Autodesk Inventor part; units mm, degrees
ref_plane "YZ Plane" through (0, 0, 0) normal (1, 0, 0) x (0, 1, 0)
ref_plane "XZ Plane" through (0, 0, 0) normal (0, 1, 0) x (-1, 0, 0)
ref_plane "XY Plane" through (0, 0, 0) normal (0, 0, 1) x (1, 0, 0)
sketch "Boceto1" plane through (0, 0, 0) normal (0, 1, 0) x (-1, 0, 0)
  circle A0 centre (0, 0) radius 9
  dimension "d0" = 18
extrude "Extrusión1" add sketch "Boceto1" along normal blind 65
sketch "Boceto2" plane through (0, 65, 0) normal (0, 1, 0) x (1, 0, 0)
  circle A0 centre (0, 0) radius 4.5
  circle A1 centre (0, 0) radius 7
  dimension "d3" = 9
  dimension "d4" = 14
extrude "Extrusión2" cut sketch "Boceto2" against normal blind 0.5
sketch "Boceto3" plane through (0, 0, 0) normal (0, -1, 0) x (1, 0, 0)
  circle A0 centre (0, 0) radius 7
extrude "Extrusión3" cut sketch "Boceto3" against normal blind 0.1
properties part number "Batería"
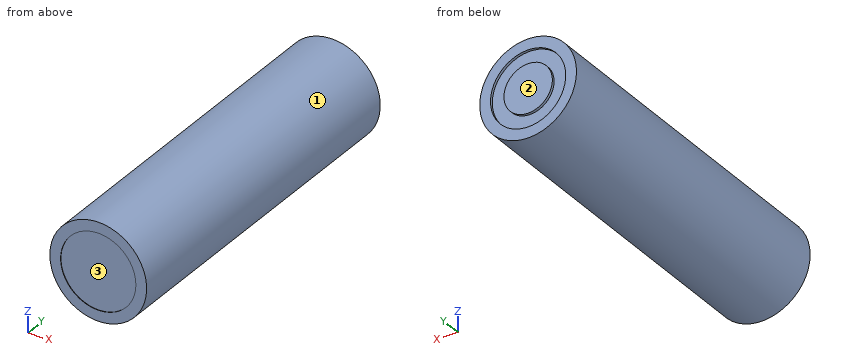
Geometry: final body of the model. Coordinates: model frame, mm. Face numbers are marked on the shaded views. Round coordinates to 2 decimals unless told otherwise and drop trailing zeros. Order: outer loops, then holes, each group sorted by start corner. A loop starts at its lowest first (then second) coordinate and runs counter-clockwise, first axis right, second up. Notation, with made-up numbers: (-16, 0.25) -> (7, 0.25) arc R31 ccw to (7, 38.25) -> close; hole circle Ø10 at (-38.75, 85). An arc over 180 degrees is marked (long way). Use one line per item in the form item = value.
(1) Draft query along Z for the marked faces 1, 2 and 3. Return one class per face: pulls with the +Z half, pulls with the -Z half, needs draft (parallel to the pull), parting line crosses it, or undercut.
Results list:
face_1 = parting line crosses it
face_2 = needs draft
face_3 = undercut
(2) First-contact query: pin 1 Ø1 at (x, y) = (1.5, 14.5) entering from +Z; pin 2 Ø5 at (y, z) = (11, -6.5) entering from +X; pin 3 Ø4 at (y, z) = (23, 4.5) entering from -X. Flat tips, straight axial feed; report the tip coordinate or a pass-through.
Results list:
pin_1 = 8.94
pin_2 = 8.06
pin_3 = -8.65
(3) Section B-B on x = 6. Return loops of the section in (y, z), and give its area (3 significant figures).
Results list:
outline = (0, -6.71) -> (65, -6.71) -> (65, -3.61) -> (64.5, -3.61) -> (64.5, 3.61) -> (65, 3.61) -> (65, 6.71) -> (0, 6.71) -> (0, 3.61) -> (0.1, 3.61) -> (0.1, -3.61) -> (0, -3.61) -> close
area = 868 mm^2
(4) Section A-A on y = 5. Return loops of the section in (x, z), and give its area (3 significant figures).
Results list:
outline = circle Ø18 at (0, 0)
area = 254 mm^2
(5) Ray query, probe 1 along Z at (x, y) = (0, 64.9); probe 2 along Z at (x, y) = (0, 0.05); probe 3 along Y at (x, z) = (0.5, -1). Return the intervals inside material, ascending. Write a range as [from, to].
Results list:
probe_1 = [-9, -7], [-4.5, 4.5], [7, 9]
probe_2 = [-9, -7], [7, 9]
probe_3 = [0.1, 65]
